from build123d import *

# Parameters (mm, degrees)
EXTRUDE_1_DEPTH     = 20
FILLET_1_R          = 2
SKETCH_2_R          = 1.5
CUT_EXTRUDE_1_DEPTH = 10


with BuildPart() as part:
    # 草图1 → 凸台-拉伸1 (new body)
    with BuildSketch(Plane(origin=(0, 0, 0), x_dir=(1, 0, 0), z_dir=(0, 1, 0))):
        with BuildLine():
            Line((0.585585586, 64.997362174), (0.495495495, 54.997767993))
            ThreePointArc((0.495495495, 54.997767993), (9.550649772, 54.164426416), (18.344731031, 51.850466183))
            Line((18.344731031, 51.850466183), (21.680136673, 61.277823671))
            ThreePointArc((21.680136673, 61.277823671), (11.287131548, 64.012503946), (0.585585586, 64.997362174))
        make_face()
    extrude(amount=EXTRUDE_1_DEPTH)

    # 圆角1
    fillet_1_edges = [part.edges().sort_by_distance(p)[0] for p in [
        (9.550649772, 0, -54.164426416),
        (0.540540541, 0, -59.997565083),
        (11.287131548, 0, -64.012503946),
        (20.012433852, 0, -56.564144927),
        (18.344731031, 10, -51.850466183),
        (0.495495495, 10, -54.997767993),
        (0.585585586, 10, -64.997362174),
        (21.680136673, 10, -61.277823671),
    ]]
    fillet(fillet_1_edges, radius=FILLET_1_R)

    # 草图2 → 切除-拉伸1 (cut)
    with BuildSketch(Plane(origin=(0, 20, 0), x_dir=(1, 0, 0), z_dir=(0, 1, 0))):
        with Locations(Location((10.111516208, 59.141840012, 0), (0, 0, 270))):
            Circle(SKETCH_2_R)
    extrude(amount=-CUT_EXTRUDE_1_DEPTH, mode=Mode.SUBTRACT)


solid = part.part
CAD build for the part. Positions are in the model's coordinates, mm. A direction names the side the tool comes from. Round coordinates to 2 decimals unless told otherwise and drop trailing zeros. Write each loop counter-clockwise with the first axis right and the second up, starting at its lowest first coordinate (ties: lowest second). Pieces come first, ordered by that corner, then holes.
(1) Slice it at A-A, the plane y = 15. Write the cut outline in (x, z), and give its area (3 significant figures).
(2) Slice it at B-B, the plane y = 3. Write the cut outline in (x, z).
(3) 3-axis set-ups, long thin cutter, end or side, ignore diameter. For faces 1 (the face through (20.918, 11.126, -60.899)), 2 (the face through (1.11, 0.6, -59.92)): which of +Z, -Z, +X, -X, +Y, -Y reach the whole face in a straight line?
(4) Mould opens along X. For faces 3 (the face through (10.56, 15.07, -57.71)), 4 (the face through (11, 0, -59)), 5 (the face through (9.452, 10.874, -54.182)), 6 (the face through (10, 10, -59)) say: pulls with the +X half, pulls with the -X half, needs draft (parallel to the pull), parting line crosses it, or undercut.
(5) Drop flat-ended pins along their axis: P1, Ø6, axis at x = 15, y = 7, coming from the -Z side; P2, Ø1.5, axis at x = 13, y = 10.5, coming from the -Z side; P3, Ø5, axis at y = 4, z = -55, coming from the +X side. Give the stop position or say it passes through.
(6) Probe line 1 along X through (y, z) = (16.75, -58.5); line 2 along Z through (x, y) = (12.75, 10); line 3 along Z through (x, y) = (6, 3.75). List the from-to ranges inside material, lowest first.
From the geometry:
1. outline: (0.51, -56.96) - (0.57, -62.97) arc R2 ccw to (2.65, -64.95) arc R65 ccw to (19.72, -61.94) arc R2 ccw to (21, -59.36) - (19, -53.7) arc R2 ccw to (16.51, -52.46) arc R55 cw to (2.42, -54.95) arc R2 ccw to start; hole circle Ø3 at (10.11, -59.14)
1. area: 188 mm2
2. outline: (0.51, -56.96) - (0.57, -62.97) arc R2 ccw to (2.65, -64.95) arc R65 ccw to (19.72, -61.94) arc R2 ccw to (21, -59.36) - (19, -53.7) arc R2 ccw to (16.51, -52.46) arc R55 cw to (2.42, -54.95) arc R2 ccw to start
3. face 1: +X, +Y, -Y
3. face 2: -Z, -X, -Y
4. face 3: undercut
4. face 4: needs draft
4. face 5: pulls with the -X half
4. face 6: undercut
5. P1: stops at z = -63.88
5. P2: stops at z = -63.84
5. P3: stops at x = 20.34
6. line 1: x = 0.53 to 8.76, 11.47 to 20.7
6. line 2: z = -63.74 to -53.5
6. line 3: z = -64.72 to -54.67
